Study the drawing (mm; zero at the part's minimum x, y, z) and answer. A direction names the side the tool comes from. Coordinates: 2 decimals unless noted, no trailing zeros. Order: outer loops, then holes, each group sorted by start corner. A loop starts at its lowest first (then second) coordinate and runs counter-clockwise, first axis right, second up. Notation, with made-up numbers: (35.5, 41.5) -> (68.5, 41.5) arc R38 ccw to (68.5, 79.5) -> close; hole circle Ø9 at (16.25, 56). An arc over 180 degrees is marked (long way). Answer in a Markdown table with one row per item. Add a question column.
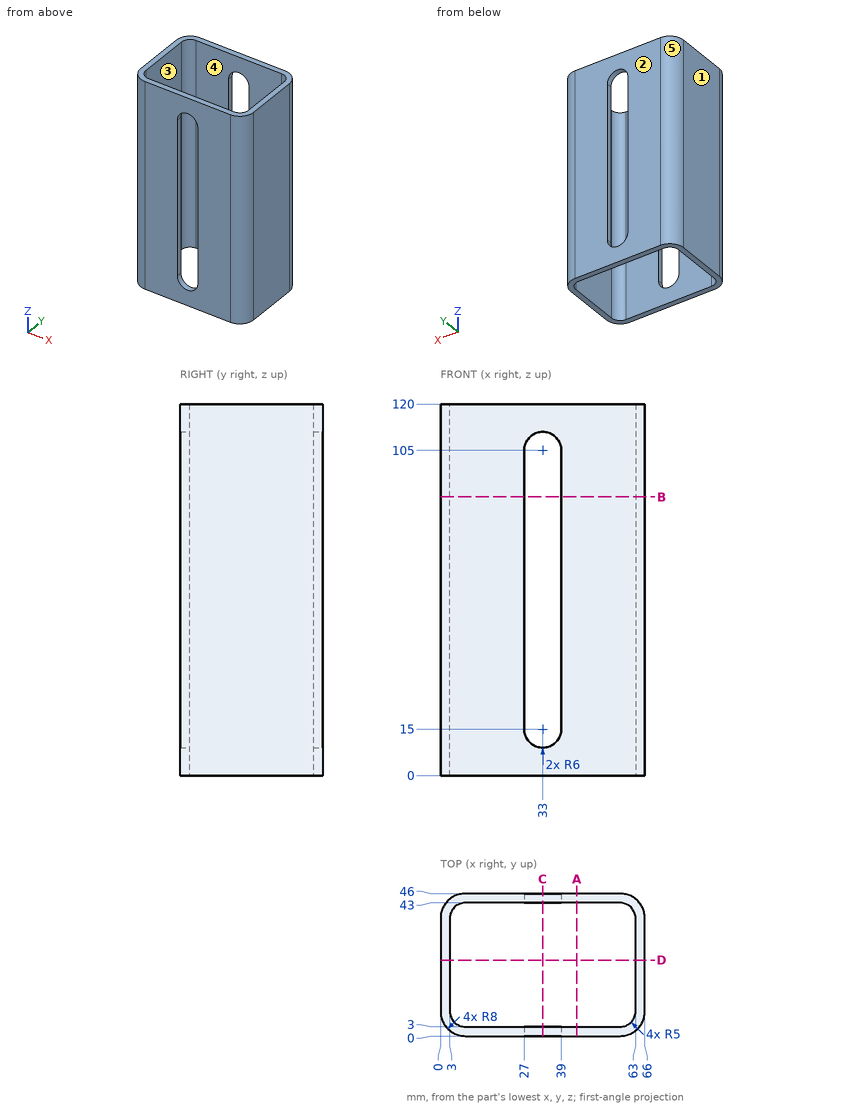
Q1. Straight lines are drawn through the part: line 1 (Y direction, x = 49.5, z = 102); line 2 (X direction, y = 28.5, z = 68.5); line 3 (X direction, y = 5, z = 103.5). For each, find the intervals that lie inside material, in ascending order.
Q2. A cutting plane is placed at B-B (z = 90). Determine the outline of the cut face in (x, y), then the cut area to 3 significant figures.
Q3. Given pin 1 (2.5 mm diameter, centred on y = 2, z = 58, fed in from +X); pin 2 (1.5 mm diameter, centred on y = 2, z = 75, fed in from -X), each flat-ended and moving along its own axis, determine where each tip first touches the part or whether it passes through.
Q4. Determine the mould class of the marked faces 1, 2 and 3 for opening direction Y: +Y half, -Y half, draft (parallel to the pull), parting line (faces both ways), or undercut.
Q5. For the marked faces 4 and 5, determine the directions among +Z, -Z, +X, -X, +Y, -Y from which every point of the face is accessible in a straight line to the end or side of a thin tool.
Q6. A cutting plane is placed at D-D (y = 24.5). Determine the outline of the cut face in (x, z), then the cut area to 3 significant figures.
Q7. A cutting plane is placed at C-C (x = 33). Determine the outline of the cut face in (y, z), then the cut area to 3 significant figures.
Q8. A cutting plane is placed at A-A (x = 44). Determine the outline of the cut face in (y, z), then the cut area to 3 significant figures.
Returned:
| question | item | result |
|---|---|---|
| 1 | line 1 | y = 0 to 3, 43 to 46 |
| 1 | line 2 | x = 0 to 3, 63 to 66 |
| 1 | line 3 | x = 0.58 to 4, 62 to 65.42 |
| 2 | outline | (0, 8) arc R8 ccw to (8, 0) -> (27, 0) -> (27, 3) -> (8, 3) arc R5 cw to (3, 8) -> (3, 38) arc R5 cw to (8, 43) -> (27, 43) -> (27, 46) -> (8, 46) arc R8 ccw to (0, 38) -> close; (39, 0) -> (58, 0) arc R8 ccw to (66, 8) -> (66, 38) arc R8 ccw to (58, 46) -> (39, 46) -> (39, 43) -> (58, 43) arc R5 cw to (63, 38) -> (63, 8) arc R5 cw to (58, 3) -> (39, 3) -> close |
| 2 | area | 531 mm² |
| 3 | pin 1 | stops at x = 64.44 |
| 3 | pin 2 | stops at x = 1.96 |
| 4 | face 1 | draft |
| 4 | face 2 | +Y half |
| 4 | face 3 | undercut |
| 5 | face 4 | +Z, -Z |
| 5 | face 5 | +Z, -Z, -X, +Y |
| 6 | outline | (0, 0) -> (3, 0) -> (3, 120) -> (0, 120) -> close; (63, 0) -> (66, 0) -> (66, 120) -> (63, 120) -> close |
| 6 | area | 720 mm² |
| 7 | outline | (0, 0) -> (3, 0) -> (3, 9) -> (0, 9) -> close; (0, 111) -> (3, 111) -> (3, 120) -> (0, 120) -> close; (43, 0) -> (46, 0) -> (46, 9) -> (43, 9) -> close; (43, 111) -> (46, 111) -> (46, 120) -> (43, 120) -> close |
| 7 | area | 108 mm² |
| 8 | outline | (0, 0) -> (3, 0) -> (3, 120) -> (0, 120) -> close; (43, 0) -> (46, 0) -> (46, 120) -> (43, 120) -> close |
| 8 | area | 720 mm² |
